Here's how the part is built. I have some questions about the finished solid (model axes, mm). Round coordinates to 2 decimals unless told otherwise and drop trailing zeros. Order: outer loops, then holes, each group sorted by start corner. A loop starts at its lowest first (then second) coordinate and runs counter-clockwise, first axis right, second up. Notation, with made-up numbers: (-32.5, 66.5) -> (16.5, 66.5) arc R20 cw to (16.5, 105.5) -> close; hole circle Ø5 at (1.5, -9). An arc over 180 degrees is marked (long way). Use a Markdown table: item, result. Add a question column.
(1) If I drill on probe 1 along Y at (x, z) = (2.5, 9); probe 2 along Y at (x, z) = (1.25, 14.5); probe 3 along X at (y, z) = (8, 14), over which ranges is the centre line in solid material (lowest first)?
(2) I want a section at B-B, the plane y = 2. Please give me the cut outline in (x, z).
(3) I want a section at D-D, the plane z = 17. Please give me the cut outline in (x, y), then the cut area to 3 significant figures.
(4) I want a section at C-C, the plane x = -0.5. Please give me the cut outline in (y, z), then the cut area to 3 significant figures.
(5) I want a section at A-A, the plane x = 2.25. Please give me the cut outline in (y, z) (3 decimals).
(6) Thinking about a two-plate mould opening in Y: for faces 1 (the face through (-4.299, 9.329, 10.704)), 2 (the face through (0, 0.25, 16)), 3 (the face through (0.171, 3.63, 13.91)), which applies, pulls with the +Y half, pulls with the -Y half, needs draft (parallel to the pull), parting line crosses it, or undercut?
(7) I'm going to push flat-ended pins straight in: P1, Ø8, axis at x = -2, y = 12.5, coming from the +Z side; P2, Ø0.5, axis at y = 4.5, z = 14, coming from the +X side; P3, Ø6, axis at y = 4, z = 12, coming from the -X side. Where does each tip first touch, or does it pass through?
from build123d import *

# Parameters (mm, degrees)
REVOLVE1_ANGLE            = 45
CUT_EXTRUDE1_DEPTH        = 28.647117169
CUT_EXTRUDE1_DEPTH_BACK   = 28.647117169
CUT_EXTRUDE4_REACH        = 29.998
CUT_EXTRUDE4_START_RADIUS = 14.22
CUT_EXTRUDE4_END_RADIUS   = 14.22
CUT_EXTRUDE5_DEPTH        = 26.131771039
CUT_EXTRUDE5_DEPTH_BACK   = 26.131771039
SKETCH9_R                 = 2.6035


with BuildPart() as part:
    # Sketch1 → Revolve1 (revolve, symmetric)
    with BuildSketch(Plane(origin=(0, 0, 0), x_dir=(0, 0, -1), z_dir=(1, 0, 0))) as revolve1_sk:
        with BuildLine():
            Line((-14.217802221, 0.25), (-19.048359509, 0.25))
            ThreePointArc((-19.048359509, 0.25), (-14.676690222, 12.144845166), (-3.81, 18.66511184))
            Line((-3.81, 18.66511184), (-3.81, 13.700083941))
            ThreePointArc((-3.81, 13.700083941), (-11.246181696, 8.70240181), (-14.217802221, 0.25))
        make_face()
    revolve(axis=Axis((0, 0, 0), (0, 1, 0)), revolution_arc=REVOLVE1_ANGLE / 2)
    revolve(revolve1_sk.sketch, axis=Axis((0, 0, 0), (0, -1, 0)), revolution_arc=REVOLVE1_ANGLE / 2)

    # Sketch2 → Cut-Extrude1 (cut, two sides: drawn at the far end of the back side and taken through both)
    with BuildSketch(Plane(origin=(0, 0, 0), x_dir=(1, 0, 0), z_dir=(0, 1, 0)).offset(-CUT_EXTRUDE1_DEPTH_BACK)):
        with BuildLine():
            Line((7.289491598, -17.598389479), (1.458023877, -3.519981019))
            ThreePointArc((1.458023877, -3.519981019), (1.400077392, -3.543428184), (1.341754023, -3.5659215))
            Line((1.341754023, -3.5659215), (7.173849701, -17.645845983))
            ThreePointArc((7.173849701, -17.645845983), (7.231709577, -17.622212591), (7.289491598, -17.598389479))
        make_face()
        with BuildLine():
            Line((-7.173849701, -17.645845983), (-1.341754023, -3.5659215))
            ThreePointArc((-1.341754023, -3.5659215), (-1.400077392, -3.543428184), (-1.458023877, -3.519981019))
            Line((-1.458023877, -3.519981019), (-7.289491598, -17.598389479))
            ThreePointArc((-7.289491598, -17.598389479), (-7.231709577, -17.622212591), (-7.173849701, -17.645845983))
        make_face()
    extrude(amount=CUT_EXTRUDE1_DEPTH + CUT_EXTRUDE1_DEPTH_BACK, mode=Mode.SUBTRACT)

    # Cut-Extrude4: from a sphere face, 29.998 long prism both ways, kept between that surface and its translate by the depth
    cut_extrude4_start = Location((0, 0, 0)) * Sphere(CUT_EXTRUDE4_START_RADIUS, mode=Mode.PRIVATE)
    cut_extrude4_end = Location((0, 0.145802388, 0.351998102)) * Sphere(CUT_EXTRUDE4_END_RADIUS, mode=Mode.PRIVATE)
    # Sketch8 → Cut-Extrude4 (cut, from a surface)
    with BuildSketch(Plane(origin=(0, 0, 0), x_dir=(-1, 0, 0), z_dir=(0, 0.3826834323650899, 0.9238795325112868)), mode=Mode.PRIVATE) as cut_extrude4_sk1:
        Polygon((-0.593913261, -0.505052528), (0.227948718, -0.505052528), (0.227948718, 3.939947472), (-0.170961538, 3.939947472), (-0.170961538, -0.049155093), (-0.854807692, -0.049155093), align=None)
    cut_extrude4_tool1 = extrude(cut_extrude4_sk1.sketch, amount=CUT_EXTRUDE4_REACH, both=True, mode=Mode.PRIVATE)
    add(((cut_extrude4_tool1 - cut_extrude4_start) & cut_extrude4_end).solids().sort_by_distance((0.031455, 4.048316, 13.618019))[0], mode=Mode.SUBTRACT)

    # Sketch9 → Cut-Extrude5 (cut, two sides: drawn at the far end of the back side and taken through both)
    with BuildSketch(Plane(origin=(0, 18.858537854, 18.858537854), x_dir=(1, 0, 0), z_dir=(0, 0.7071067811865478, 0.7071067811865474)).offset(-CUT_EXTRUDE5_DEPTH_BACK)):
        with Locations(Location((0, 0, 0), (0, 0, 90))):
            Circle(SKETCH9_R)
    extrude(amount=CUT_EXTRUDE5_DEPTH + CUT_EXTRUDE5_DEPTH_BACK, mode=Mode.SUBTRACT)


solid = part.part
Taken from the geometry:
| question | item | result |
|---|---|---|
| 1 | probe 1 | y = 10.72 to 16.6 |
| 1 | probe 2 | y = 0.25 to 11.27 |
| 1 | probe 3 | x = -5.66 to 5.66 |
| 2 | outline | (-7.13, 17.55) -> (-5.27, 13.05) arc R14.08 cw to (-0.23, 14.08) -> (-0.23, 14.45) arc R14.1 cw to (0.17, 14.45) -> (0.17, 14.08) arc R14.08 cw to (5.27, 13.05) -> (7.13, 17.55) arc R18.94 ccw to start |
| 3 | outline | (-6.91, 0.25) -> (6.91, 0.25) -> (6.91, 5.12) arc R8.6 ccw to (-6.91, 5.12) -> close |
| 3 | area | 101 mm2 |
| 4 | outline | (0.25, 14.21) arc R14.21 cw to (8.08, 11.69) -> (11.54, 15.15) arc R19.04 ccw to (0.25, 19.04) -> close; (11.69, 8.08) arc R14.21 cw to (13.7, 3.78) -> (18.67, 3.78) arc R19.04 ccw to (15.15, 11.54) -> close |
| 4 | area | 81.8 mm2 |
| 5 | outline | (0.25, 14.039) arc R14.041 cw to (8.959, 10.811) -> (12.418, 14.27) arc R18.917 ccw to (0.25, 18.915) -> close; (10.811, 8.959) arc R14.041 cw to (12.806, 5.759) -> (18.019, 5.759) arc R18.917 ccw to (14.27, 12.418) -> close |
| 6 | face 1 | needs draft |
| 6 | face 2 | pulls with the -Y half |
| 6 | face 3 | undercut |
| 7 | P1 | stops at z = 16.97 |
| 7 | P2 | stops at x = 5.77 |
| 7 | P3 | stops at x = -6.08 |
